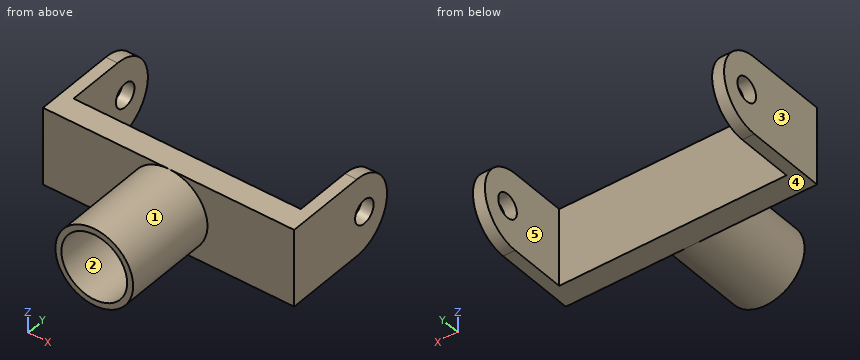
from build123d import *

# Parameters (mm, degrees)
SKETCH1_R               = 3.25
SKETCH1_R_2             = 2.75
BOSS_EXTRUDE1_DEPTH     = 8
SKETCH2_W               = 21
SKETCH2_H               = 6.5
BOSS_EXTRUDE2_DEPTH     = 2
SKETCH3_W               = 1
SKETCH3_H               = 6.5
BOSS_EXTRUDE3_DEPTH     = 8
CUT_EXTRUDE1_DEPTH      = 28.84892278
CUT_EXTRUDE1_DEPTH_BACK = 28.84892278
SKETCH4_R               = 1
FILLET1_RADIUS          = 3.25
FILLET1_LENGTH          = 1
FILLET2_RADIUS          = 3.25
FILLET2_LENGTH          = 1


with BuildPart() as part:
    # Sketch1 → Boss-Extrude1 (new body)
    with BuildSketch(Plane(origin=(0, 0, 0), x_dir=(1, 0, 0), z_dir=(0, 1, 0))):
        with Locations(Location((0, 0, 0), (0, 0, 270))):
            Circle(SKETCH1_R)
        with Locations(Location((0, 0, 0), (0, 0, 270))):
            Circle(SKETCH1_R_2, mode=Mode.SUBTRACT)
    extrude(amount=BOSS_EXTRUDE1_DEPTH)

    # Sketch2 → Boss-Extrude2 (add)
    with BuildSketch(Plane(origin=(0, 8, 0), x_dir=(1, 0, 0), z_dir=(0, 1, 0))):
        Rectangle(SKETCH2_W, SKETCH2_H)
    extrude(amount=BOSS_EXTRUDE2_DEPTH)

    # Sketch3 → Boss-Extrude3 (add)
    with BuildSketch(Plane(origin=(0, 10, 0), x_dir=(1, 0, 0), z_dir=(0, 1, 0))):
        with Locations((-10, 0)):
            Rectangle(SKETCH3_W, SKETCH3_H)
        with Locations((10, 0)):
            Rectangle(SKETCH3_W, SKETCH3_H)
    extrude(amount=BOSS_EXTRUDE3_DEPTH)

    # Sketch4 → Cut-Extrude1 (cut, two sides: drawn at the far end of the back side and taken through both)
    with BuildSketch(Plane.ZY.offset(10.5).offset(-CUT_EXTRUDE1_DEPTH_BACK)):
        with Locations((0, 15.56)):
            Circle(SKETCH4_R)
    extrude(amount=CUT_EXTRUDE1_DEPTH + CUT_EXTRUDE1_DEPTH_BACK, mode=Mode.SUBTRACT)

    # Fillet1: full round fillet: the end face becomes a half cylinder, R = half its width
    fillet1_face = Plane((10, 18, 0), x_dir=(-1, 0, 0), z_dir=(0, 1, 0))  # on the end face: x along it, z out of the body
    fillet1_slab = fillet1_face.offset(-FILLET1_RADIUS / 2) * Box(FILLET1_LENGTH, 2 * FILLET1_RADIUS, FILLET1_RADIUS, mode=Mode.PRIVATE)  # the body's end, R deep
    fillet1_round = Plane((10, 14.75, 0), x_dir=(0, 1, 0), z_dir=(-1, 0, 0)) * Cylinder(FILLET1_RADIUS, FILLET1_LENGTH, mode=Mode.PRIVATE)  # its axis R under the face
    add(fillet1_slab - fillet1_round, mode=Mode.SUBTRACT)

    # Fillet2: full round fillet: the end face becomes a half cylinder, R = half its width
    fillet2_face = Plane((-10, 18, 0), x_dir=(1, 0, 0), z_dir=(0, 1, 0))  # on the end face: x along it, z out of the body
    fillet2_slab = fillet2_face.offset(-FILLET2_RADIUS / 2) * Box(FILLET2_LENGTH, 2 * FILLET2_RADIUS, FILLET2_RADIUS, mode=Mode.PRIVATE)  # the body's end, R deep
    fillet2_round = Plane((-10, 14.75, 0), x_dir=(0, 1, 0), z_dir=(1, 0, 0)) * Cylinder(FILLET2_RADIUS, FILLET2_LENGTH, mode=Mode.PRIVATE)  # its axis R under the face
    add(fillet2_slab - fillet2_round, mode=Mode.SUBTRACT)


solid = part.part
Could you check a few things on this model? Use its own coordinates, in mm. Face numbers are marked on the shaded views. A direction names the side the tool comes from. Give positions to 0.01 mm unless a question says otherwise; leave off trailing zeros. Loops run counter-clockwise (first coordinate to the right, second up) from the corner with the lowest first, then second, coordinate; pieces in that order, holes last. Notation, with made-up numbers: (-5, 78.25) -> (44, 78.25) arc R28 ccw to (44, 110.25) -> close; hole circle Ø5 at (-13.75, 68). An arc over 180 degrees is marked (long way). Return JSON: item names as keys, results as strings.
Item 1: If we section it at B-B on y = 15.56: List the corners of the cut face in (x, z) for me.
Geometry results:
{"outline": "(-10.5, -3.15) -> (-9.5, -3.15) -> (-9.5, -1) -> (-10.5, -1) -> close; (-10.5, 1) -> (-9.5, 1) -> (-9.5, 3.15) -> (-10.5, 3.15) -> close; (9.5, -3.15) -> (10.5, -3.15) -> (10.5, -1) -> (9.5, -1) -> close; (9.5, 1) -> (10.5, 1) -> (10.5, 3.15) -> (9.5, 3.15) -> close"}
Item 2: I'm going to push flat-ended pins straight in: pin 1 (1.5 mm diameter, centred on y = 5, z = 0, fed in from +X); pin 2 (2 mm diameter, centred on x = 5, y = 2.5, fed in from -Z); pin 3 (3 mm diameter, centred on x = 1, z = 0.5, fed in from -Y). Where does each tip first touch, or does it pass through?
Geometry results:
{"pin 1": "stops at x = 3.25", "pin 2": "passes through", "pin 3": "stops at y = 8"}
Item 3: If we section it at D-D on y = 5.25: List the corners of the cut face in (x, z) for me, plus the area to 3 significant figures.
Geometry results:
{"outline": "circle Ø6.5 at (0, 0); hole circle Ø5.5 at (0, 0)", "area": "9.42 mm²"}
Item 4: I need wall thicknesses on L1, parallel to X at y = 12.5, z = -3; L2, parallel to Y at x = -10.2, z = 0; L3, parallel to X at y = 6.25, z = 0. Which ranges of each line are inside material? Lowest first, please. Write a range as from..to.
Geometry results:
{"L1": "x = -10.5..-9.5, 9.5..10.5", "L2": "y = 8..14.56, 16.56..18", "L3": "x = -3.25..-2.75, 2.75..3.25"}
Item 5: If we section it at A-A on z = 0: List the corners of the cut face in (x, y) for me, plus the area to 3 significant figures.
Geometry results:
{"outline": "(-10.5, 8) -> (-3.25, 8) -> (-3.25, 0) -> (-2.75, 0) -> (-2.75, 8) -> (2.75, 8) -> (2.75, 0) -> (3.25, 0) -> (3.25, 8) -> (10.5, 8) -> (10.5, 14.56) -> (9.5, 14.56) -> (9.5, 10) -> (-9.5, 10) -> (-9.5, 14.56) -> (-10.5, 14.56) -> close; (-10.5, 16.56) -> (-9.5, 16.56) -> (-9.5, 18) -> (-10.5, 18) -> close; (9.5, 16.56) -> (10.5, 16.56) -> (10.5, 18) -> (9.5, 18) -> close", "area": "62.0 mm²"}
Item 6: If we section it at C-C on z = -1.5: List the corners of the cut face in (x, y) for me.
Geometry results:
{"outline": "(-10.5, 8) -> (-2.88, 8) -> (-2.88, 0) -> (-2.3, 0) -> (-2.3, 8) -> (2.3, 8) -> (2.3, 0) -> (2.88, 0) -> (2.88, 8) -> (10.5, 8) -> (10.5, 17.63) -> (9.5, 17.63) -> (9.5, 10) -> (-9.5, 10) -> (-9.5, 17.63) -> (-10.5, 17.63) -> close"}
Item 7: Which directions (+Z, -Z, +X, -X, +Y, -Y) give clear straight access to the entire face, cutting with the end or side of a thin tool? Please do the marked faces 4 and 5.
Geometry results:
{"face 4": "-Z, +X, -X, +Y, -Y", "face 5": "+Z, -Z, +Y"}
Item 8: We'd pull the mould along X, two halves only. Please class the marked faces 1, 2 and 3: +X half, -X half, draft (parallel to the pull), parting line (faces both ways), or undercut.
Geometry results:
{"face 1": "parting line", "face 2": "undercut", "face 3": "-X half"}
